The listing builds one solid part. Answer for the finished solid, in the listing's coordinates (mm). Round coordinates to 2 decimals unless told otherwise and drop trailing zeros. Loops run counter-clockwise (first coordinate to the right, second up) from the corner with the lowest first, then second, coordinate; pieces in that order, holes last. Notation, with made-up numbers: M -29,70 L -17,70 A7 ccw -17,83 Z; hole C -37.75,67 d6. An arc over 180 degrees is marked long. Put each result on its own line as item: value. Start each with the question number.
(1) Section A-A, the plane x = 140.5 is taken. Determine the outline of the cut face in (y, z).
(2) Flat-ended cylindrical pins translate along their axes: P1, Ø3.5, axis at x = 31.5, z = 7.5, coming from the -Y side; P2, Ø2, axis at x = 67.5, y = -130, coming from the -Z side; P3, Ø0.7, axis at x = -169, z = 7.5, coming from the +Y side; P4, Ø4.5, axis at x = 3.5, y = -117.5, coming from the +Z side. Find the tip coordinate at first contact, or state that the pin passes through.
(3) Straight lines are drawn through the part: line 1 (X direction, y = -123, z = 7.5); line 2 (Z direction, x = -163, y = -124.25); line 3 (X direction, y = -124.75, z = 9). For each, find the intervals that lie inside material, in ascending order.
```python
from build123d import *

# Parameters (mm, degrees)
F0_R     = 2
F1_DEPTH = 16
F2_SIZE  = 2
F3_W     = 349
F3_H     = 16
F4_DEPTH = 3.1
F5_W     = 345.2
F5_H     = 5
F6_DEPTH = 12
F7_R     = 2
F8_DEPTH = 17.272573


with BuildPart() as f1:
    # F0 (on Top) → F1 (new body)
    with BuildSketch(Plane.XY):
        with BuildLine():
            Line((-171.5, -127.73274), (-171.5, -131.223399))
            Line((-171.5, -131.223399), (171.5, -131.223399))
            Line((171.5, -131.223399), (171.5, -127.73274))
            Line((171.5, -127.73274), (171.5, -118.223399))
            ThreePointArc((171.5, -118.223399), (170.914214, -116.809185), (169.5, -116.223399))
            Line((169.5, -116.223399), (168.828427, -116.223399))
            ThreePointArc((168.828427, -116.223399), (168.06306, -116.071158), (167.414214, -115.637612))
            Line((167.414214, -115.637612), (164.414214, -112.637612))
            ThreePointArc((164.414214, -112.637612), (163, -112.051826), (161.585786, -112.637612))
            Line((161.585786, -112.637612), (158.585786, -115.637612))
            ThreePointArc((158.585786, -115.637612), (157.93694, -116.071158), (157.171573, -116.223399))
            Line((157.171573, -116.223399), (-154.5, -116.223399))
            Line((-154.5, -116.223399), (-157.171573, -116.223399))
            ThreePointArc((-157.171573, -116.223399), (-157.93694, -116.071158), (-158.585786, -115.637612))
            Line((-158.585786, -115.637612), (-161.585786, -112.637612))
            ThreePointArc((-161.585786, -112.637612), (-163, -112.051826), (-164.414214, -112.637612))
            Line((-164.414214, -112.637612), (-167.414214, -115.637612))
            ThreePointArc((-167.414214, -115.637612), (-168.06306, -116.071158), (-168.828427, -116.223399))
            Line((-168.828427, -116.223399), (-169.5, -116.223399))
            ThreePointArc((-169.5, -116.223399), (-170.914214, -116.809185), (-171.5, -118.223399))
            Line((-171.5, -118.223399), (-171.5, -127.73274))
        make_face()
        with Locations((-114.333, -121.723399)):
            Circle(F0_R, mode=Mode.SUBTRACT)
        with Locations((0, -121.723399)):
            Circle(F0_R, mode=Mode.SUBTRACT)
        with Locations((114.333, -121.723399)):
            Circle(F0_R, mode=Mode.SUBTRACT)
    extrude(amount=F1_DEPTH)

    # F2
    f2_edges = [f1.edges().sort_by_distance(p)[0] for p in [
        (0, -131.223399, 16),
    ]]
    chamfer(f2_edges, length=F2_SIZE)

    # F3 (on face) → F4 (cut)
    with BuildSketch(Plane.XY.offset(16)):
        with Locations((0, -119.223399)):
            Rectangle(F3_W, F3_H)
    extrude(amount=-F4_DEPTH, mode=Mode.SUBTRACT)

    # F5 (on face) → F6 (cut)
    with BuildSketch(Plane.XY):
        with Locations((0, -131.823399)):
            Rectangle(F5_W, F5_H)
    extrude(amount=F6_DEPTH, mode=Mode.SUBTRACT)

    # F7 (on face) → F8 (cut, through all)
    with BuildSketch(Plane.XZ.offset(129.323399)):
        with Locations((-163, 8)):
            Circle(F7_R)
        with Locations((163, 8)):
            Circle(F7_R)
    extrude(amount=-F8_DEPTH, mode=Mode.SUBTRACT)


solid = f1.part
```
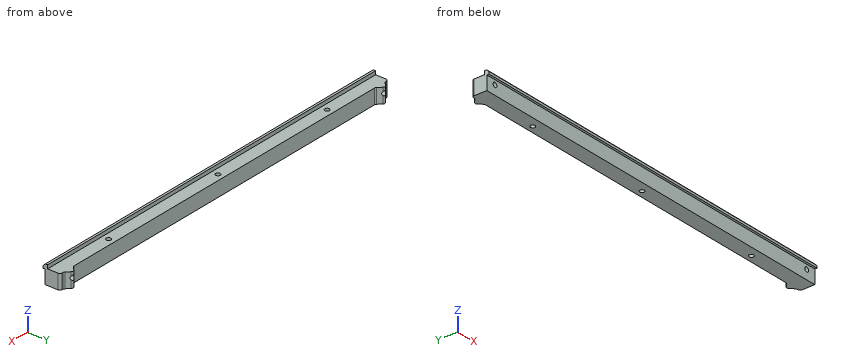
Recorded:
1. outline: M -131.22,12 L -129.32,12 L -129.32,0 L -116.22,0 L -116.22,12.9 L -127.22,12.9 L -127.22,16 L -129.22,16 L -131.22,14 Z
2. P1: stops at y = -129.32
2. P2: stops at z = 0
2. P3: stops at y = -116.22
2. P4: stops at z = 12.9
3. line 1: x = -171.5 to -164.94, -161.06 to -115.87, -112.79 to -1.54, 1.54 to 112.79, 115.87 to 161.06, 164.94 to 171.5
3. line 2: z = 0 to 6, 10 to 12.9
3. line 3: x = -171.5 to -164.73, -161.27 to 161.27, 164.73 to 171.5
